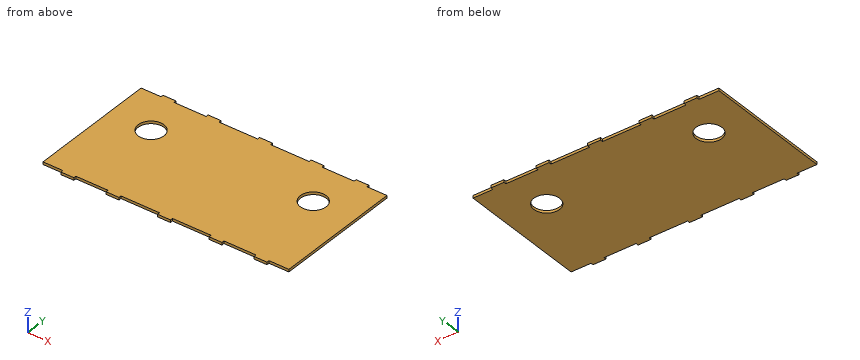
Solid Edge part; units mm, degrees
sketch "Sketch1" plane through (0, 0, 0) normal (0, 0, 1) x (1, 0, 0)
  line L0 (-160, 104) -> (-160, 100)
  line L1 (-160, 100) -> (-191, 100)
  line L2 (-191, 100) -> (-191, -100)
  line L3 (-191, -100) -> (-160, -100)
  line L4 (-160, -100) -> (-160, -104)
  line L5 (-160, -104) -> (-140, -104)
  line L6 (-140, -104) -> (-140, -100)
  line L7 (-140, -100) -> (-90, -100)
  line L8 (-90, -100) -> (-90, -104)
  line L9 (-90, -104) -> (-70, -104)
  line L10 (-70, -104) -> (-70, -100)
  line L11 (-70, -100) -> (-10, -100)
  line L12 (-10, -100) -> (-10, -104)
  line L13 (-10, -104) -> (10, -104)
  line L14 (10, -104) -> (10, -100)
  line L15 (10, -100) -> (70, -100)
  line L16 (70, -100) -> (70, -104)
  line L17 (70, -104) -> (90, -104)
  line L18 (90, -104) -> (90, -100)
  line L19 (90, -100) -> (140, -100)
  line L20 (140, -100) -> (140, -104)
  line L21 (140, -104) -> (160, -104)
  line L22 (160, -104) -> (160, -100)
  line L23 (160, -100) -> (191, -100)
  line L24 (191, -100) -> (191, 100)
  line L25 (191, 100) -> (160, 100)
  line L26 (160, 100) -> (160, 104)
  line L27 (160, 104) -> (140, 104)
  line L28 (140, 104) -> (140, 100)
  line L29 (140, 100) -> (90, 100)
  line L30 (90, 100) -> (90, 104)
  line L31 (90, 104) -> (70, 104)
  line L32 (70, 104) -> (70, 100)
  line L33 (70, 100) -> (10, 100)
  line L34 (10, 100) -> (10, 104)
  line L35 (10, 104) -> (-10, 104)
  line L36 (-10, 104) -> (-10, 100)
  line L37 (-10, 100) -> (-70, 100)
  line L38 (-70, 100) -> (-70, 104)
  line L39 (-70, 104) -> (-90, 104)
  line L40 (-90, 104) -> (-90, 100)
  line L41 (-90, 100) -> (-140, 100)
  line L42 (-140, 100) -> (-140, 104)
  line L43 (-140, 104) -> (-160, 104)
  circle A0 centre (126, 35) radius 20
  circle A1 centre (-126, 35) radius 20
extrude "Protrusion1" add sketch "Sketch1" along normal blind 4
Model file for the job. Use its own axes, mm. Give positions to 0.01 mm unless a question says otherwise; leave off trailing zeros. Loops run counter-clockwise (first coordinate to the right, second up) from the corner with the lowest first, then second, coordinate; pieces in that order, holes last. Notation, with made-up numbers: (-33.5, 37.25) - (-22.5, 37.25) arc R26 ccw to (-22.5, 62.25) - close; hole circle Ø11 at (66, 88). An arc over 180 degrees is marked (long way). One line per item, written item: value. Start each with the question number.
1. Slice it at D-D (x = -65.5). List the corners of the cut face in (y, z), plus the area to 3 significant figures.
2. Slice it at A-A (x = 126). List the corners of the cut face in (y, z).
3. Probe L1, parallel to Y at x = -126, z = 2.75; L2, parallel to Y at x = -31.5, z = 1.75; L3, parallel to Y at x = 112.5, z = 3.25. List the from-to ranges inside material, lowest first. Write a range as from..to.
4. Pin check, flat tips, straight feed: pin 1 (2 mm diameter, centred on y = -102, z = 2, fed in from +X); pin 2 (1.2 mm diameter, centred on y = -103, z = 1, fed in from -X); pin 3 (2 mm diameter, centred on x = -32, z = 2.5, fed in from +Y). Stop position of each tip, or through.
5. Slice it at C-C (z = 1.2). Give the number of separate pieces and of enclosed holes in the cut face, plus the area to 3 significant figures.
6. Slice it at B-B (y = 35). List the corners of the cut face in (x, z), plus the area to 3 significant figures.
Solution:
1. outline: (-100, 0) - (100, 0) - (100, 4) - (-100, 4) - close
1. area: 800 mm^2
2. outline: (-100, 0) - (15, 0) - (15, 4) - (-100, 4) - close; (55, 0) - (100, 0) - (100, 4) - (55, 4) - close
3. L1: y = -100..15, 55..100
3. L2: y = -100..100
3. L3: y = -100..20.24, 49.76..100
4. pin 1: stops at x = 160
4. pin 2: stops at x = -160
4. pin 3: stops at y = 100
5. separate pieces: 1
5. enclosed holes: 2
5. area: 74,700 mm^2
6. outline: (-191, 0) - (-146, 0) - (-146, 4) - (-191, 4) - close; (-106, 0) - (106, 0) - (106, 4) - (-106, 4) - close; (146, 0) - (191, 0) - (191, 4) - (146, 4) - close
6. area: 1,210 mm^2
